from build123d import *

# Parameters (mm, degrees)
SKETCH1_R           = 12
SKETCH1_R_2         = 14
SKETCH1_R_3         = 10
SKETCH1_R_4         = 7
BOSS_EXTRUDE1_DEPTH = 5


with BuildPart() as part:
    # Sketch1 → Boss-Extrude1 (new, symmetric)
    with BuildSketch(Plane.XY):
        with BuildLine():
            ThreePointArc((11, 88), (0, 99), (-11, 88))
            Line((-11, 88), (-22, 88))
            ThreePointArc((-22, 88), (-26.70940007, 58.656200039), (-49, 39))
            ThreePointArc((-49, 39), (-68.998392946, 18.746465817), (-48.492972379, -0.993572042))
            ThreePointArc((-48.492972379, -0.993572042), (-39.014510451, -3.809523143), (-33.001122743, -11.658726248))
            ThreePointArc((-33.001122743, -11.658726248), (-28.18429152, -20.752004999), (-20.931196761, -28.051470588))
            ThreePointArc((-20.931196761, -28.051470588), (-14.77228566, -37.934411824), (-16.94430214, -49.375))
            ThreePointArc((-16.94430214, -49.375), (-9.320242105, -77.695566877), (18.346551197, -67.962666587))
            Line((18.346551197, -67.962666587), (38.567256581, -67.962666587))
            ThreePointArc((38.567256581, -67.962666587), (54.123605767, -61.519015773), (60.567256581, -45.962666587))
            Line((60.567256581, -45.962666587), (67.180494628, 16.984907625))
            ThreePointArc((67.180494628, 16.984907625), (63.971087494, 29.810935932), (53.255704219, 37.556118792))
            ThreePointArc((53.255704219, 37.556118792), (27.844090476, 56.715909688), (22, 88))
            Line((22, 88), (11, 88))
        make_face()
        with Locations((0, -60)):
            Circle(SKETCH1_R, mode=Mode.SUBTRACT)
        Circle(SKETCH1_R_2, mode=Mode.SUBTRACT)
        with BuildLine():
            Line((34.793024979, 3.800712147), (37, 19))
            ThreePointArc((37, 19), (48, 30), (59, 19))
            ThreePointArc((59, 19), (58.885841276, 17.419348327), (58.545734598, 15.871504867))
            Line((58.545734598, 15.871504867), (49.567256581, -45.962666587))
            ThreePointArc((49.567256581, -45.962666587), (38.567256581, -56.962666587), (27.567256581, -45.962666587))
            ThreePointArc((27.567256581, -45.962666587), (27.681415305, -44.382014914), (28.021521984, -42.834171454))
            Line((28.021521984, -42.834171454), (34.793024979, 3.800712147))
        make_face(mode=Mode.SUBTRACT)
        with Locations((-49, 19)):
            Circle(SKETCH1_R_3, mode=Mode.SUBTRACT)
        with Locations((0, 88)):
            Circle(SKETCH1_R_4, mode=Mode.SUBTRACT)
    extrude(amount=BOSS_EXTRUDE1_DEPTH, both=True)


solid = part.part
Design review of the part built by this model. Coordinates are the model's own, in mm. A direction names the side the tool comes from. Round coordinates to 2 decimals unless told otherwise and drop trailing zeros. Write each loop counter-clockwise with the first axis right and the second up, starting at its lowest first coordinate (ties: lowest second). Pieces come first, ordered by that corner, then holes. Notation, with made-up numbers: (60.25, -18.75) - (97.25, -18.75) arc R24 cw to (97.25, 11.25) - close; hole circle Ø7 at (24, 16.25). An arc over 180 degrees is marked (long way). Return JSON: item names as keys, results as strings. Group by question number.
Item 1: We need section A-A on x = 0. Write out the cut boundary in (y, z).
Item 2: The part is to be moulded in two halves that separate along X. For faces 1 (the face through (54.12, -14.61, 0.07)), 2 (the face through (13, 11, 5)), 3 (the face through (64.08, 29.65, 0.07)), 4 (the face through (0, 99, 0)), say which applies: pulls with the +X half, pulls with the -X half, needs draft (parallel to the pull), parting line crosses it, or undercut.
Item 3: We need section C-C on y = 27. Write out the cut boundary in (x, z).
Item 4: For probe 1 along Y at (x, z) = (0, 0); probe 2 along X at (y, z) = (13, -1.5); probe 3 along Y at (x, z) = (-49, -3), list the stretches that pass through material, from the lowest coordinate up. Write a range as [from, to].
Item 5: We need section B-B on y = -60. Write out the cut boundary in (x, z), and give its area (3 significant figures).
Item 6: Insertion check: P1, Ø5, axis at x = 25.5, z = 0, coming from the -Y side; P2, Ø3, axis at x = 18, z = 1.5, coming from the +Y side; P3, Ø6, axis at y = -27, z = -3, coming from the +X side. Each pin has a flat end and moves straight along its axis. Give the tip position at first contact, or say it passes through.
Item 7: We need section D-D on z = -2.5. Write out the cut boundary in (x, y) (1 decimal).
Item 8: Machinability: for faces 5 (the face through (17, 88, 0)), 6 (the face through (28.086, 56.33, 0.07)), 7 (the face through (28, -67.963, 0)), which of the approach directions +Z, -Z, +X, -X, +Y, -Y give a long, thin tool a straight path to every point of the face, cutting with its end or side? Answer none if there is none.
Model answer:
{
 "1": {"outline": "(-80, -5) - (-72, -5) - (-72, 5) - (-80, 5) - close; (-48, -5) - (-14, -5) - (-14, 5) - (-48, 5) - close; (14, -5) - (81, -5) - (81, 5) - (14, 5) - close; (95, -5) - (99, -5) - (99, 5) - (95, 5) - close"},
 "2": {"face 1": "undercut", "face 2": "needs draft", "face 3": "pulls with the +X half", "face 4": "parting line crosses it"},
 "3": {"outline": "(-67.33, -5) - (-55, -5) - (-55, 5) - (-67.33, 5) - close; (-43, -5) - (40.45, -5) - (40.45, 5) - (-43, 5) - close; (55.55, -5) - (65.55, -5) - (65.55, 5) - (55.55, 5) - close"},
 "4": {"probe 1": "y = [-80, -72], [-48, -14], [14, 81], [95, 99]", "probe 2": "x = [-68.08, -57], [-41, -5.2], [5.2, 36.13], [58.13, 66.76]", "probe 3": "y = [-1, 9], [29, 39]"},
 "5": {"outline": "(-20, -5) - (-12, -5) - (-12, 5) - (-20, 5) - close; (12, -5) - (55.51, -5) - (55.51, 5) - (12, 5) - close", "area": "515 mm²"},
 "6": {"P1": "stops at y = -67.96", "P2": "stops at y = 88", "P3": "stops at x = 62.87"},
 "7": {"outline": "(-49, 39) arc R20 ccw (long way) to (-48.5, -1) arc R16 cw to (-33, -11.7) arc R35 ccw to (-20.9, -28.1) arc R16 cw to (-16.9, -49.4) arc R20 ccw (long way) to (18.3, -68) - (38.6, -68) arc R22 ccw to (60.6, -46) - (67.2, 17) arc R19.3 ccw to (53.3, 37.6) arc R44 cw to (22, 88) - (11, 88) arc R11 ccw to (-11, 88) - (-22, 88) arc R44 cw to start; hole circle Ø20 at (-49, 19); hole circle Ø28 at (0, 0); hole circle Ø24 at (0, -60); hole circle Ø14 at (0, 88); hole (28, -42.8) arc R11 ccw (long way) to (49.6, -46) - (58.5, 15.9) arc R11 ccw (long way) to (37, 19) - close"},
 "8": {"face 5": "+Z, -Z, +X, +Y", "face 6": "+Z, -Z, +X", "face 7": "+Z, -Z, +X, -Y"}
}
